Here's how the part is built. I have some questions about the finished solid (model axes, mm). Face numbers are marked on the shaded views. A direction names the side the tool comes from. Round coordinates to 2 decimals unless told otherwise and drop trailing zeros. Order: outer loops, then holes, each group sorted by start corner. A loop starts at its lowest first (then second) coordinate and runs counter-clockwise, first axis right, second up.
```python
from build123d import *

# Parameters (mm, degrees)
FURO_ROSCADO_DE_M12X1_51_D           = 10.5
FURO_ROSCADO_DE_M12X1_51_DEPTH       = 41.5
FURO_ROSCADO_DE_M12X1_51_CSINK_D     = 12.05
FURO_ROSCADO_DE_M12X1_51_CSINK_ANGLE = 90
FURO_ROSCADO_DE_M12X1_51_TIP         = 3.15451825
FURO1_D                              = 9.8
FURO1_DEPTH                          = 25
CHANFRO1_SIZE                        = 1
CHANFRO3_SIZE                        = 1
FILETE1_R                            = 0.5
CHANFRO4_SIZE                        = 0.5


with BuildPart() as part:
    # Esboço1 → Revolução1 (revolve)
    with BuildSketch(Plane.XY, mode=Mode.PRIVATE) as revolu_o1_sk:
        Polygon((0, 0), (65, 0), (65, 11), (55, 11), (55, 9.25), (50, 9.25), (50, 11), (5, 11), (5, 9.25), (0, 9.25), align=None)
    revolve(revolu_o1_sk.sketch.rotate(Axis((0, 0, 0), (1, 0, 0)), 90), axis=Axis((0, 0, 0), (1, 0, 0)))

    # Furo roscado de M12x1.51
    with Locations(Plane(origin=(65, 0, 0), x_dir=(0, 0, -1), z_dir=(1, 0, 0))):
        with Locations((0, 0)):
            CounterSinkHole(FURO_ROSCADO_DE_M12X1_51_D / 2, FURO_ROSCADO_DE_M12X1_51_CSINK_D / 2, depth=FURO_ROSCADO_DE_M12X1_51_DEPTH, counter_sink_angle=FURO_ROSCADO_DE_M12X1_51_CSINK_ANGLE)
            with Locations((0, 0, -(FURO_ROSCADO_DE_M12X1_51_DEPTH + FURO_ROSCADO_DE_M12X1_51_TIP / 2))):  # 118° drill point
                Cone(0, FURO_ROSCADO_DE_M12X1_51_D / 2, FURO_ROSCADO_DE_M12X1_51_TIP, mode=Mode.SUBTRACT)

    # Furo1
    with Locations(Plane.ZY):
        with Locations((0, 0)):
            Hole(FURO1_D / 2, depth=FURO1_DEPTH)

    # Chanfro1
    chanfro1_edges = [part.edges().sort_by_distance(p)[0] for p in [
        (5, 0, -11),
    ]]
    chamfer(chanfro1_edges, length=CHANFRO1_SIZE)

    # Chanfro3
    chanfro3_edges = [part.edges().sort_by_distance(p)[0] for p in [
        (50, 0, -11),
    ]]
    chamfer(chanfro3_edges, length=CHANFRO3_SIZE)

    # Filete1
    filete1_edges = [part.edges().sort_by_distance(p)[0] for p in [
        (65, 0, -11),
        (0, 0, -9.25),
        (55, 0, -11),
    ]]
    fillet(filete1_edges, radius=FILETE1_R)

    # Chanfro4
    chanfro4_edges = [part.edges().sort_by_distance(p)[0] for p in [
        (0, 0, 4.9),
    ]]
    chamfer(chanfro4_edges, length=CHANFRO4_SIZE)


solid = part.part
```
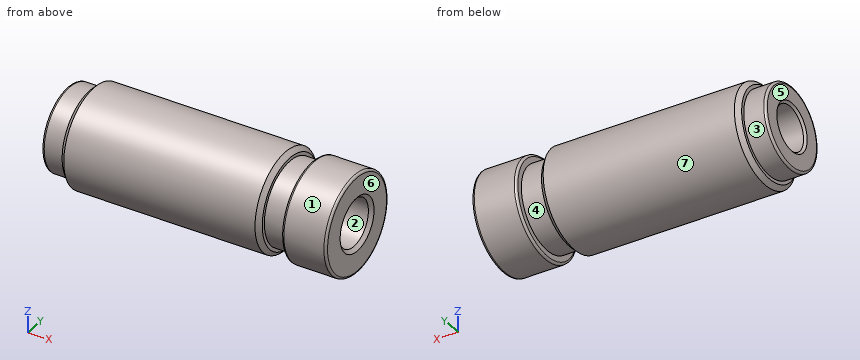
1. If we section it at B-B, the plane x = 18.5: Write out the boundary of the cut face in (y, z).
Evaluation:
outline: circle Ø22 at (0, 0); hole circle Ø9.8 at (0, 0)
2. I'm going to push flat-ended pins straight in: P1, Ø12, axis at y = 0, z = 0, coming from the +X side (3 decimals); P2, Ø12, axis at x = 12, z = -7.5, coming from the -Y side; P3, Ø8, axis at x = 29, z = -7.5, coming from the +Y side. Where does each tip first touch, or does it pass through?
Evaluation:
P1: stops at x = 64.975
P2: stops at y = -10.9
P3: stops at y = 10.43
3. If we mould it in two halves opening along X, with no side actions, what happens to the marked faces 4, 5, 6 and 7? For each: released by +X, released by -X, zero draft, split by the parting line, or undercut.
Evaluation:
face 4: undercut
face 5: released by -X
face 6: released by +X
face 7: zero draft
4. I need wall thicknesses on probe 1 along Y at (x, z) = (6, 0); probe 2 along X at (y, z) = (8.75, 1.25); probe 3 along X at (y, z) = (-6.5, 8.5). Which ranges of each line are inside material? Lowest first, please.
Evaluation:
probe 1: y = -11 to -4.9, 4.9 to 11
probe 2: x = 0.01 to 65
probe 3: x = 5.7 to 49.3, 55.04 to 64.96
5. If we section it at A-A, the plane x = 29: Write out the boundary of the cut face in (y, z).
Evaluation:
outline: circle Ø22 at (0, 0); hole circle Ø10.5 at (0, 0)
6. On a 3-axis mill with a long thin cutter (end or side, diameter ignored), from which of +Z, -Z, +X, -X, +Y, -Y can I reach the whole of each face in a straight line? I mean the marked faces 1, 2 and 3. Say none if no direction works.
Evaluation:
face 1: +X, -X
face 2: +X
face 3: -X
